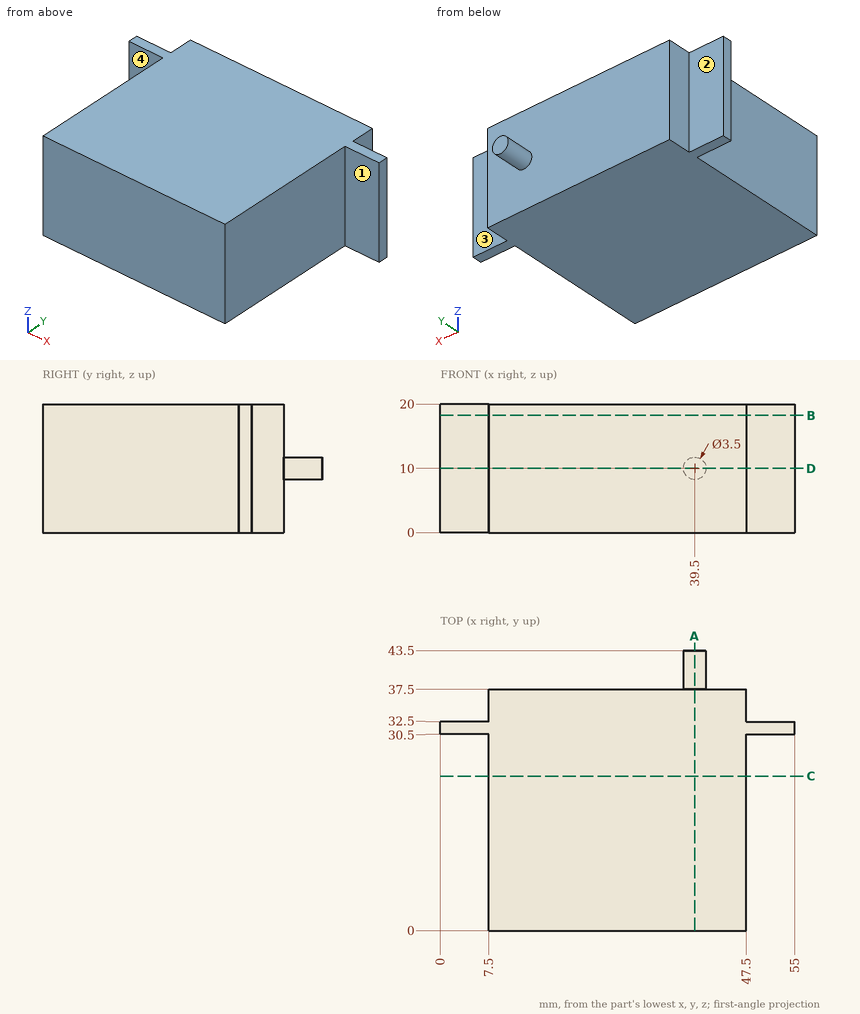
Geometry check sheet. Reference: drawing and pictorial views, mm from the part's lowest x, y, z. A direction names the side the tool comes from. Round coordinates to 2 decimals unless told otherwise and drop trailing zeros. Loops run counter-clockwise (first coordinate to the right, second up) from the corner with the lowest first, then second, coordinate; pieces in that order, holes last. Notation, with made-up numbers: (-13, 41) - (24, 41) arc R31 cw to (24, 72) - close; hole circle Ø9 at (67, -23). An arc over 180 degrees is marked (long way). Answer in a Markdown table with one row per item. Add a question column.
Q1. Gauge pin test, flat ends, axial feed: pin 1 (1.5 mm diameter, centred on y = 8, z = 18, fed in from +X); pin 2 (10 mm diameter, centred on x = 22, z = 8, fed in from +Y); pin 3 (6 mm diameter, centred on x = 51.5, z = 11.5, fed in from +Y). Record the tip position at first contact, or that the pin passes through.
Q2. Section check B-B on z = 18.25. Enter the section's corners in (x, y).
Q3. Section check A-A on x = 39.5. Enter the section's corners in (y, z).
Q4. Tool access check on the marked faces 1, 2, 3 and 4. Record the directions out of +Z, -Z, +X, -X, +Y, -Y that give a thin tool (end or side, any length) a straight path to the whole face; none if there is none.
Q5. Section check C-C on y = 24. Enter the section's corners in (x, z), plus the area to 3 significant figures.
Q6. Section check D-D on z = 10. Enter the section's corners in (x, y), plus the area to 3 significant figures.
Q7. Material ranges on line 1 (X direction, y = 33, z = 8.5); line 2 (Y direction, x = 41, z = 11.5); line 3 (Y direction, x = 4, z = 5.75), recorded low to high.
Found:
| question | item | result |
|---|---|---|
| 1 | pin 1 | stops at x = 47.5 |
| 1 | pin 2 | stops at y = 37.5 |
| 1 | pin 3 | stops at y = 32.5 |
| 2 | outline | (0, 30.5) - (7.5, 30.5) - (7.5, 0) - (47.5, 0) - (47.5, 30.5) - (55, 30.5) - (55, 32.5) - (47.5, 32.5) - (47.5, 37.5) - (7.5, 37.5) - (7.5, 32.5) - (0, 32.5) - close |
| 3 | outline | (0, 0) - (37.5, 0) - (37.5, 8.25) - (43.5, 8.25) - (43.5, 11.75) - (37.5, 11.75) - (37.5, 20) - (0, 20) - close |
| 4 | face 1 | +Z, -Z, +X, -Y |
| 4 | face 2 | +Z, -Z, -X, +Y |
| 4 | face 3 | +Z, -Z, +X, +Y |
| 4 | face 4 | +Z, -Z, -X, -Y |
| 5 | outline | (7.5, 0) - (47.5, 0) - (47.5, 20) - (7.5, 20) - close |
| 5 | area | 800 mm² |
| 6 | outline | (0, 30.5) - (7.5, 30.5) - (7.5, 0) - (47.5, 0) - (47.5, 30.5) - (55, 30.5) - (55, 32.5) - (47.5, 32.5) - (47.5, 37.5) - (41.25, 37.5) - (41.25, 43.5) - (37.75, 43.5) - (37.75, 37.5) - (7.5, 37.5) - (7.5, 32.5) - (0, 32.5) - close |
| 6 | area | 1,550 mm² |
| 7 | line 1 | x = 7.5 to 47.5 |
| 7 | line 2 | y = 0 to 37.5 |
| 7 | line 3 | y = 30.5 to 32.5 |
